from build123d import *

# Parameters (mm, degrees)
SKETCH1_R               = 50
BOSS_EXTRUDE1_DEPTH     = 60
BOSS_EXTRUDE1_TAPER     = 15
CUT_EXTRUDE1_DEPTH      = 140.28388293
CUT_EXTRUDE1_DEPTH_BACK = 140.28388293
SKETCH2_R               = 25


with BuildPart() as part:
    # Sketch1 → Boss-Extrude1 (new body)
    with BuildSketch(Plane(origin=(0, 0, 0), x_dir=(1, 0, 0), z_dir=(0, 1, 0))):
        Circle(SKETCH1_R)
    boss_extrude1 = extrude(amount=BOSS_EXTRUDE1_DEPTH, taper=BOSS_EXTRUDE1_TAPER)

    # Mirror2: Boss-Extrude1 across plane
    add(boss_extrude1.mirror(Plane.ZX.offset(60)))

    # Sketch2 → Cut-Extrude1 (cut, two sides: drawn at the far end of the back side and taken through both)
    with BuildSketch(Plane(origin=(0, 120, 0), x_dir=(1, 0, 0), z_dir=(0, 1, 0)).offset(-CUT_EXTRUDE1_DEPTH_BACK)):
        with Locations(Location((0, 0, 0), (0, 0, 270))):
            Circle(SKETCH2_R)
    extrude(amount=CUT_EXTRUDE1_DEPTH + CUT_EXTRUDE1_DEPTH_BACK, mode=Mode.SUBTRACT)


solid = part.part
Could you check a few things on this model? Use its own coordinates, in mm. A direction names the side the tool comes from. Give positions to 0.01 mm unless a question says otherwise; leave off trailing zeros. Order: outer loops, then holes, each group sorted by start corner. A loop starts at its lowest first (then second) coordinate and runs counter-clockwise, first axis right, second up. Notation, with made-up numbers: (42, 55.5) - (59, 55.5) arc R20 ccw to (59, 87.5) - close; hole circle Ø4 at (-6.75, 53). An arc over 180 degrees is marked (long way). One line per item, written item: value. Start each with the question number.
1. Imagine slicing it at B-B on y = 92.5. List the corners of the cut face in (x, z) for me, plus the area to 3 significant figures.
2. Thinking about a two-plate mould opening in Z: for faces 3 (the face through (35.36, 76.25, 14.66)), 4 (the face through (7.509, 59.16, 23.846)), 5 (the face through (-22.9, 120, 10.4)), which applies, +Z half, -Z half, draft (parallel to the pull), parting line (faces both ways), or undercut?
3. For P1, Ø1, axis at y = 44, z = -5.5, coming from the -X side; P2, Ø3, axis at y = 61, z = -12.5, coming from the -X side; P3, Ø4, axis at y = 81, z = 33.5, coming from the +X side; P4, Ø12, axis at x = 27.5, z = -18, coming from the -Y side, each with a flat end and sliding along its axis, tell me the tip position at first contact or that it passes through.
4. Imagine slicing it at A-A on x = 0. List the corners of the cut face in (y, z) for me, plus the area to 3 significant figures.
5. If I drill on probe 1 along X at (y, z) = (55.5, -12); probe 2 along Z at (x, y) = (0.5, 35) (3 decimals); probe 3 along X at (y, z) = (36.5, 18), over which ranges is the centre line in solid material (lowest first)?
6. Imagine slicing it at C-C on y = 109. List the corners of the cut face in (x, z) for me.
7. For faces 1 (the face through (36.51, 43.75, -11.5)), 2 (the face through (-22.9, 0, 10.4)), which set-ups out of +Z, -Z, +X, -X, +Y, -Y let a thin tool reach every point of the face, with its end or its side?
Values:
1. outline: circle Ø85.26 at (0, 0); hole circle Ø50 at (0, 0)
1. area: 3,750 mm²
2. face 3: parting line
2. face 4: undercut
2. face 5: draft
3. P1: x = -37.97
3. P2: x = -32.53
3. P3: x = 24.06
3. P4: y = 0
4. outline: (0, -50) - (60, -33.92) - (120, -50) - (120, -25) - (0, -25) - close; (0, 25) - (120, 25) - (120, 50) - (60, 33.92) - (0, 50) - close
4. area: 4,070 mm²
5. probe 1: -33.02 to -21.93, 21.93 to 33.02
5. probe 2: -40.619 to -24.995, 24.995 to 40.619
5. probe 3: -35.97 to -17.35, 17.35 to 35.97
6. outline: circle Ø94.11 at (0, 0); hole circle Ø50 at (0, 0)
7. face 1: none
7. face 2: +Z, -Z, +X, -X, -Y
